For this review, take the finished solid that the model builds, in its own axes (mm). Face numbers are marked on the shaded views. Give positions to 0.01 mm unless a question says otherwise; leave off trailing zeros. Loops run counter-clockwise (first coordinate to the right, second up) from the corner with the lowest first, then second, coordinate; pieces in that order, holes last.
```python
from build123d import *

# Parameters (mm, degrees)
SKETCH1_W           = 105
SKETCH1_H           = 105
BOSS_EXTRUDE1_DEPTH = 20
HOLE5_OUTLINE_R     = 40
HOLE5_DEPTH         = 20
SKETCH14_R          = 5
CUT_EXTRUDE2_DEPTH  = 20
LPATTERN2_COUNT     = 2
LPATTERN2_PITCH     = 30
FILLET3_R           = 50


# Read off the part's stored shape, not the designer's step: Hole5
with BuildPart() as part:
    # Sketch1 → Boss-Extrude1 (new body)
    with BuildSketch(Plane(origin=(-15.357562319, 50.523240315, 0), x_dir=(1, 0, 0), z_dir=(0, 0, 1))):
        with Locations((-36.920942408, -46.377068063)):
            Rectangle(SKETCH1_W, SKETCH1_H)
    extrude(amount=BOSS_EXTRUDE1_DEPTH)

    # Hole5 outline → Hole5 (cut)
    with BuildSketch(Plane.XY):
        with Locations((-52.692198598, -3.343760422)):
            Circle(HOLE5_OUTLINE_R)
    extrude(amount=HOLE5_DEPTH, mode=Mode.SUBTRACT)

    # Sketch14 → Cut-Extrude2 (cut)
    with BuildSketch(Plane(origin=(0, 0, 0), x_dir=(-1, 0, 0), z_dir=(0, 0, -1))):
        with Locations((37.278504727, 49.646172252)):
            Circle(SKETCH14_R)
    cut_extrude2 = extrude(amount=-CUT_EXTRUDE2_DEPTH, mode=Mode.SUBTRACT)

    # LPattern2: Cut-Extrude2 ×2
    with Locations(*[(-i * LPATTERN2_PITCH, 0, 0) for i in range(1, LPATTERN2_COUNT)]):
        add(cut_extrude2, mode=Mode.SUBTRACT)

    # Fillet3
    fillet3_edges = [part.edges().sort_by_distance(p)[0] for p in [
        (-104.778504727, 56.646172252, 10),
        (0.221495273, 56.646172252, 10),
        (0.221495273, -48.353827748, 10),
        (-104.778504727, -48.353827748, 10),
    ]]
    fillet(fillet3_edges, radius=FILLET3_R)


solid = part.part
```
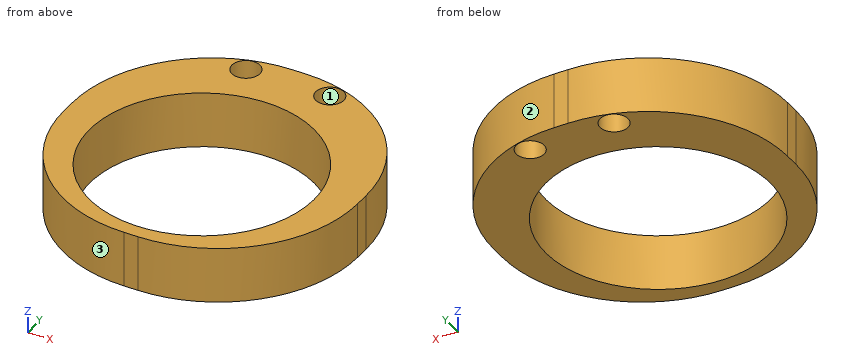
Q1. Consider section B-B on y = 13.5. Give the boundary of the cut face in (x, z), plus the area to 3 significant figures.
Answers:
outline: (-104.31, 0) - (-88.97, 0) - (-88.97, 20) - (-104.31, 20) - close; (-16.41, 0) - (-0.25, 0) - (-0.25, 20) - (-16.41, 20) - close
area: 630 mm2
Q2. Consider section A-A on x = -17. Give the boundary of the cut face in (y, z), plus the area to 3 significant figures.
Answers:
outline: (-36.11, 0) - (-21.4, 0) - (-21.4, 20) - (-36.11, 20) - close; (14.71, 0) - (44.4, 0) - (44.4, 20) - (14.71, 20) - close
area: 888 mm2
Q3. Consider section C-C on z = 5.5. Give the boundary of the cut face in (x, y), plus the area to 3 significant figures.
Answers:
outline: (-104.78, 1.65) arc R50 ccw to (-54.78, -48.35) - (-49.78, -48.35) arc R50 ccw to (0.22, 1.65) - (0.22, 6.65) arc R50 ccw to (-49.78, 56.65) - (-54.78, 56.65) arc R50 ccw to (-104.78, 6.65) - close; hole circle Ø80 at (-52.69, -3.34); hole circle Ø10 at (-67.28, 49.65); hole circle Ø10 at (-37.28, 49.65)
area: 3,700 mm2
Q4. For probe 1 along X at (y, z) = (52, 15.75); probe 2 along Y at (x, z) = (-41, 8); probe 3 along Y at (x, z) = (-72.5, 5.25), list the stretches that pass through material, from the lowest coordinate up.
Answers:
probe 1: x = -75.83 to -71.69, -62.87 to -41.69, -32.87 to -28.73
probe 2: y = -47.58 to -41.6, 34.91 to 46.31, 52.99 to 55.87
probe 3: y = -45.11 to -38.1, 31.41 to 53.4
Q5. For pin 1 Ø12 at (x, z) = (-82, 13) entering from +Y; pin 2 Ø1 at (y, z) = (40.5, 16) entering from -X; pin 3 Ø10 at (x, z) = (-93.5, 17.5) entering from +Y; pin 4 Ø5 at (x, y) = (-21, -20.5) entering from -Z, all flat-tipped, find the tip position at first contact; note any pin that passes through.
Answers:
pin 1: stops at y = 51.92
pin 2: stops at x = -92.03
pin 3: stops at y = 43.56
pin 4: passes through
Q6. Mouldability with a two-part tool opening along X and no side actions: class the marked faces 1, 2 and 3 as +X half, -X half, draft (parallel to the pull), parting line (faces both ways), or undercut.
Answers:
face 1: undercut
face 2: +X half
face 3: -X half
